CAD build for the part. Positions are in the model's coordinates, mm. Face numbers are marked on the shaded views. A direction names the side the tool comes from. Give positions to 0.01 mm unless a question says otherwise; leave off trailing zeros. Write each loop counter-clockwise with the first axis right and the second up, starting at its lowest first coordinate (ties: lowest second). Pieces come first, ordered by that corner, then holes. Notation, with made-up numbers: (22, 77.5) -> (67, 77.5) arc R21 ccw to (67, 112.5) -> close; hole circle Ø3 at (-1, 88). An arc over 180 degrees is marked (long way). Answer as a JSON object with one key per item and string values.
```python
from build123d import *

# Parameters (mm, degrees)
CHAMFER1_SIZE      = 0.5
CUT_EXTRUDE1_DEPTH = 2.5


with BuildPart() as part:
    # Sketch1 → Revolve1 (revolve)
    with BuildSketch(Plane.XY):
        Polygon((-5, 0), (10, 0), (10, 2.5), (0, 2.5), (0, 4.25), (-5, 4.25), align=None)
    revolve(axis=Axis((-5, 0, 0), (1, 0, 0)))

    # Chamfer1
    chamfer1_edges = [part.edges().sort_by_distance(p)[0] for p in [
        (-5, -4.25, 0),
    ]]
    chamfer(chamfer1_edges, length=CHAMFER1_SIZE)

    # Sketch2 → Cut-Revolve1 (revolve, cut)
    with BuildSketch(Plane.XY):
        Polygon((-1.298278762, 0), (-2.5, 2), (-5, 2), (-5, 0), align=None)
    revolve(axis=Axis((-5, 0, 0), (1, 0, 0)), mode=Mode.SUBTRACT)

    # Sketch3 → Cut-Extrude1 (cut)
    with BuildSketch(Plane.ZY.offset(5)):
        Polygon((0, -2.309401077), (2, -1.154700538), (2, 1.154700538), (0, 2.309401077), (-2, 1.154700538), (-2, -1.154700538), align=None)
    extrude(amount=-CUT_EXTRUDE1_DEPTH, mode=Mode.SUBTRACT)


solid = part.part
```
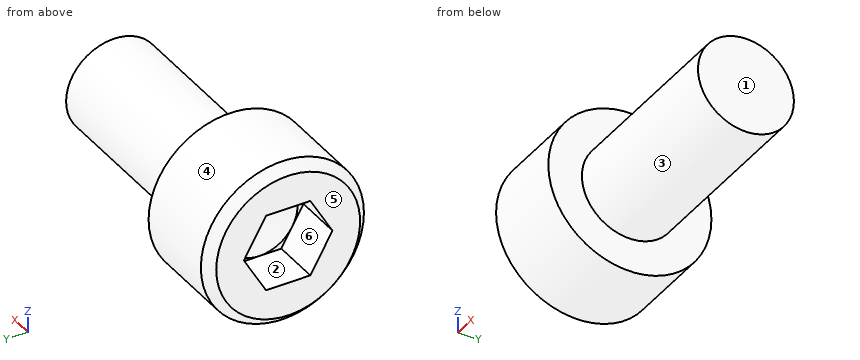
1) Wall check: probe 1 along Z at (x, y) = (-2.5, -3.75); probe 2 along X at (y, z) = (-1, 3); probe 3 along Y at (x, z) = (-0.75, 2). Give the ranges that are in metal, low to high.
Model answer:
{"probe 1": "z = -2 to 2", "probe 2": "x = -5 to 0", "probe 3": "y = -3.75 to 3.75"}
2) Slice it at A-A (x = 8.5). List the corners of the cut face in (y, z), then the cut area to 3 significant figures.
Model answer:
{"outline": "circle Ø5 at (0, 0)", "area": "19.6 mm2"}
3) Mould opens along Y. For the marked faces 4, 5 and 6 say: released by +Y, released by -Y, zero draft, split by the parting line, or undercut.
Model answer:
{"face 4": "split by the parting line", "face 5": "zero draft", "face 6": "undercut"}
4) 3-axis set-ups, long thin cutter, end or side, ignore diameter. For the marked faces 1, 2 and 3: which of +Z, -Z, +X, -X, +Y, -Y reach the whole face in a straight line?
Model answer:
{"face 1": "+Z, -Z, +X, +Y, -Y", "face 2": "-X", "face 3": "+X"}
5) Pin check, flat tip, straight feed: pin 1 (2 mm diameter, centred on x = 3.5, y = -1, fed in from -Z). Stop position of the tip, or through.
Model answer:
{"pin 1": "stops at z = -2.5"}
